Autodesk Inventor part; units mm, degrees
ref_plane "YZ Plane" through (0, 0, 0) normal (1, 0, 0) x (0, 1, 0)
ref_plane "XZ Plane" through (0, 0, 0) normal (0, 1, 0) x (-1, 0, 0)
ref_plane "XY Plane" through (0, 0, 0) normal (0, 0, 1) x (1, 0, 0)
sketch "Sketch1" plane through (0, 0, 0) normal (0, 1, 0) x (-1, 0, 0)
  line L0 (0, 0) -> (85.48, 0)
  line L1 (85.48, 0) -> (85.48, -127.76)
  line L2 (85.48, -127.76) -> (0, -127.76)
  line L3 (0, -127.76) -> (0, 0)
  line L4 (85.48, 0) -> (67.5195, -17.9605)
  line L5 (85.48, 0) -> (110.88, 0) construction
  line L6 (0, 0) -> (17.9605, -17.9605)
  line L7 (85.48, -127.76) -> (67.5195, -109.7995)
  line L8 (85.48, -127.76) -> (110.88, -127.76) construction
  line L9 (0, -127.76) -> (17.9605, -109.7995)
  line L10 (0, -127.76) -> (25.4, -127.76) construction
  dimension "d0" = 85.48
  dimension "d1" = 127.76
  dimension "d2" = 25.4
  dimension "d3" = 135
  dimension "d4" = 25.4
  dimension "d5" = 25.4
  dimension "d6" = 135
  dimension "d7" = 25.4
  dimension "d8" = 45
extrude "Extrusion1" add sketch "Sketch1" along normal blind 47.7
sketch "Sketch2" plane through (0, 0, 0) normal (0, -1, 0) x (1, 0, 0)
  line L0 (-85.48, 0) -> (0, 0)
  line L1 (0, 0) -> (-17.9605, -17.9605)
  line L2 (0, 0) -> (25.4, 0) construction
  line L3 (0, 0) -> (0, -127.76)
  line L4 (0, -127.76) -> (-17.9605, -109.7995)
  line L5 (0, -127.76) -> (25.4, -127.76) construction
  line L6 (-85.48, -127.76) -> (-85.48, 0)
  line L7 (-85.48, 0) -> (-67.5195, -17.9605)
  line L8 (-85.48, 0) -> (-60.08, 0) construction
  line L9 (0, -127.76) -> (-85.48, -127.76)
  line L10 (-85.48, -127.76) -> (-67.5195, -109.7995)
  line L11 (-85.48, -127.76) -> (-60.08, -127.76) construction
  dimension "d11" = 25.4
  dimension "d12" = 135
  dimension "d13" = 25.4
  dimension "d14" = 135
  dimension "d15" = 25.4
  dimension "d16" = 45
  dimension "d17" = 25.4
  dimension "d18" = 45
hole "Hole1" at (-17.9605, 0, -17.9605) at (-67.5195, 0, -17.9605) at (-67.5195, 0, -109.7995) at (-17.9605, 0, -109.7995) direction (0, 1, 0) diameter 3.683 depth 9.525 tip angle 118
sketch "Sketch4" plane through (0, 47.7, 0) normal (0, 1, 0) x (1, 0, 0)
  line L0 (0, -1.0521) -> (19.05, -1.0521) construction
  line L1 (0, 0) -> (0, 127.76)
  line L2 (0, 18.3507) -> (0, 0)
  line L3 (0, 0) -> (-18.7946, 0)
  line L4 (0, 0) -> (-17.3355, 0)
  line L5 (-17.3355, 0) -> (-17.3355, 13.1191)
  line L6 (-17.3355, 13.1191) -> (0, 13.1191)
  line L7 (0, 13.1191) -> (0, 0)
  dimension "d41" = 17.3355
  dimension "d42" = 13.1191
hole "Hole2" at (-17.3355, 47.7, -13.1191) direction (0, -1, 0) diameter 21 depth 35
pattern_linear "Rectangular Pattern1" count 3 spacing 25.4 along (-1, 0, 0) count 5 spacing 25.4 along (0, 0, -1) of "Hole2"
sketch "Sketch5" plane through (-85.48, 0, -127.76) normal (-1, 0, 0) x (0, 0, 1)
  line L0 (127.76, 0) -> (127.76, 47.7)
  line L1 (127.76, 0) -> (89.66, 0)
  line L2 (89.66, 0) -> (89.66, 6.35)
  line L3 (89.66, 6.35) -> (127.76, 6.35)
  line L4 (127.76, 6.35) -> (127.76, 0)
  line L5 (62.646, 6.35) -> (127.76, 6.35)
  line L6 (127.76, 6.35) -> (127.76, 0)
  line L7 (127.76, 0) -> (62.646, 0)
  line L8 (62.646, 0) -> (62.646, 6.35)
  dimension "d43" = 38.1
  dimension "d44" = 6.35
hole "Hole3" at (-85.48, 6.35, -38.1) direction (1, 0, 0) diameter 6.35 depth 31.75 tip angle 118
sketch "Sketch6" plane through (-85.48, 0, -127.76) normal (-1, 0, 0) x (0, 0, 1)
  line L0 (61.854, 6.5465) -> (127.76, 6.5465)
  line L1 (127.76, 6.5465) -> (127.76, 0.1965)
  line L2 (127.76, 0.1965) -> (61.854, 0.1965)
  line L3 (61.854, 0.1965) -> (61.854, 6.5465)
  point P0 (127.76, 0)
  dimension "d52" = 6.35
hole "Hole4" at (-85.48, 6.5465, -65.906) direction (1, 0, 0) diameter 3.175 depth 50.8 tip angle 118
sketch "Sketch7" plane through (0, 0, 0) normal (1, 0, 0) x (0, 0, -1)
  line L0 (127.76, 0) -> (0, 0)
  line L1 (127.76, 0) -> (89.66, 0)
  line L2 (89.66, 0) -> (89.66, 6.35)
  line L3 (89.66, 6.35) -> (127.76, 6.35)
  line L4 (127.76, 6.35) -> (127.76, 0)
  dimension "d60" = 38.1
  dimension "d61" = 6.35
hole "Hole5" at (0, 6.35, -89.66) direction (-1, 0, 0) diameter 6.35 depth 31.75 tip angle 118
properties part number "Thermal_topplate_5mL"
Geometry check sheet. Reference: the model listing, model coordinates, mm. A direction names the side the tool comes from. Coordinates: 2 decimals unless noted, no trailing zeros. Order: outer loops, then holes, each group sorted by start corner. A loop starts at its lowest first (then second) coordinate and runs counter-clockwise, first axis right, second up. Notation, with made-up numbers: M 77,-3.5 L 119,-3.5 A12 cw 119,5.5 Z; hole C -12.75,79.5 d11. An arc over 180 degrees is marked long. Use CSV: the item, a comma, the result in double quotes.
Item 1: Mould release check, pull along X, two halves, no side actions. Record for faces 1 (the flat face through (-85.48, 24, -63)), 2 (the flat face through (-42, 0, -63)), 3 (the conical face through (-17.86, 10.44, -110.1)): pulls with the +X half, pulls with the -X half, needs draft (parallel to the pull), parting line crosses it, or undercut.
Returned:
face 1,"pulls with the -X half"
face 2,"needs draft"
face 3,"undercut"
Item 2: Cross-section at C-C on y = 23.5. Give the number of separate pieces and of enclosed holes in the cut face, then the cut area to 3 significant figures.
Returned:
separate pieces,"1"
enclosed holes,"15"
area,"5,730 mm2"
Item 3: Thickness scan on line 1 along Z through (x, y) = (-43.5, 45); line 2 along X through (y, z) = (34.5, -62); line 3 along Z through (x, y) = (-37, 35.5). Record the ranges inside material, lowest first.
Returned:
line 1,"z = -127.76 to -125.19, -104.25 to -99.79, -78.85 to -74.39, -53.45 to -48.99, -28.05 to -23.59, -2.65 to 0"
line 2,"x = -85.48 to -78.46, -57.81 to -53.06, -32.41 to -27.66, -7.01 to 0"
line 3,"z = -127.76 to -123.51, -105.92 to -98.11, -80.52 to -72.71, -55.12 to -47.31, -29.72 to -21.91, -4.32 to 0"
Item 4: Cross-section at D-D on x = -36. Record the cut outline in (y, z) (1 decimal).
Returned:
outline,"M 0,-127.8 L 47.7,-127.8 L 47.7,-122.8 L 12.7,-122.8 L 12.7,-106.7 L 47.7,-106.7 L 47.7,-97.4 L 12.7,-97.4 L 12.7,-81.3 L 47.7,-81.3 L 47.7,-72 L 12.7,-72 L 12.7,-55.9 L 47.7,-55.9 L 47.7,-46.6 L 12.7,-46.6 L 12.7,-30.5 L 47.7,-30.5 L 47.7,-21.2 L 12.7,-21.2 L 12.7,-5.1 L 47.7,-5.1 L 47.7,0 L 0,0 Z; hole C 6.5,-65.9 d3.2"
Item 5: Cross-section at A-A on x = -21.5. Record the cut outline in (y, z) (3 decimals), then the cut area to 3 significant figures.
Returned:
outline,"M 0,-127.76 L 47.7,-127.76 L 47.7,-124.358 L 12.7,-124.358 L 12.7,-105.08 L 47.7,-105.08 L 47.7,-98.958 L 12.7,-98.958 L 12.7,-79.68 L 47.7,-79.68 L 47.7,-73.558 L 12.7,-73.558 L 12.7,-54.28 L 47.7,-54.28 L 47.7,-48.158 L 12.7,-48.158 L 12.7,-28.88 L 47.7,-28.88 L 47.7,-22.758 L 12.7,-22.758 L 12.7,-3.48 L 47.7,-3.48 L 47.7,0 L 0,0 Z; hole C 6.35,-89.66 d6.35"
area,"2,690 mm2"
Item 6: Tool access check on faces 4 (the cylindrical face through (-17.255, 4.829, -19.662)), 5 (the flat face through (-68, 12.7, -115)). Record the directions out of +Z, -Z, +X, -X, +Y, -Y that give a thin tool (end or side, any length) a straight path to the whole face; none if there is none.
Returned:
face 4,"-Y"
face 5,"+Y"
Item 7: Cross-section at B-B on z = -81. Record the cut outline in (x, y).
Returned:
outline,"M -85.48,0 L 0,0 L 0,47.7 L -10.93,47.7 L -10.93,12.7 L -23.74,12.7 L -23.74,47.7 L -36.33,47.7 L -36.33,12.7 L -49.14,12.7 L -49.14,47.7 L -61.73,47.7 L -61.73,12.7 L -74.54,12.7 L -74.54,47.7 L -85.48,47.7 Z"
Item 8: Gauge pin test, flat ends, axial feed: pin 1 Ø19 at (x, z) = (-68.14, -13.12) entering from +Y; pin 2 Ø5.5 at (y, z) = (6.35, -89.66) entering from +X. Record the tip position at first contact, or that the pin passes through.
Returned:
pin 1,"stops at y = 12.7"
pin 2,"stops at x = -32.01"
